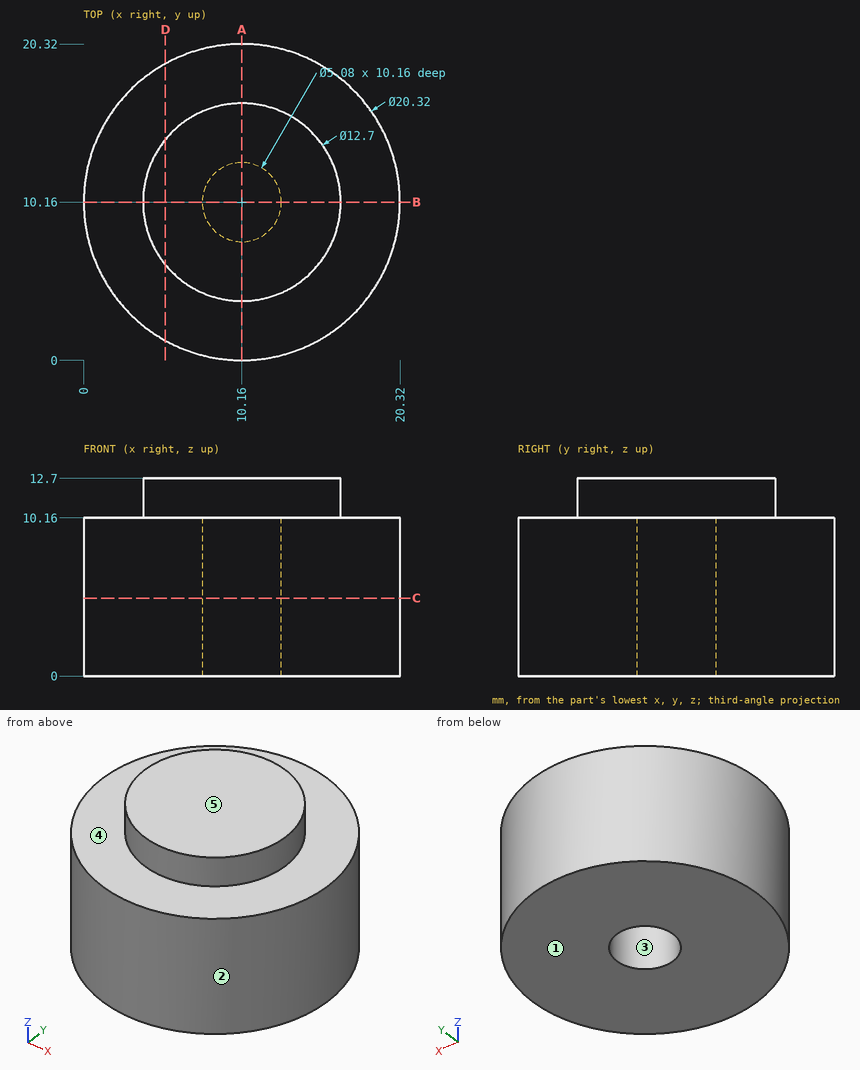
Verification items for this drawing (mm, ordinates from the low corner). A direction names the side the tool comes from. Give positions to 0.01 mm unless a question says otherwise; leave off trailing zeros. Write each loop counter-clockwise with the first axis right and the second up, starting at its lowest first coordinate (ties: lowest second). Pieces come first, ordered by that corner, then holes. Notation, with made-up numbers: (-21.75, -13) -> (-13.75, -13) arc R27 cw to (-13.75, 6) -> close; hole circle Ø8 at (67, 65.25). An arc over 180 degrees is marked (long way). Write item = value, one per line.
Item 1: Scan lines: probe 1 along Y at (x, z) = (10.16, 7.75); probe 2 along X at (y, z) = (10, 1.25); probe 3 along Z at (x, y) = (8.75, 19.5). Record each from-to range of solid material in increasing order. Write a range as from..to.
Output:
probe_1 = 0..7.62, 12.7..20.32
probe_2 = 0..7.63, 12.69..20.32
probe_3 = 0..10.16
Item 2: Sectioned sample at C-C on z = 5. Record the boundary of the cut face in (x, y).
Output:
outline = circle Ø20.32 at (10.16, 10.16); hole circle Ø5.08 at (10.16, 10.16)
Item 3: Sectioned sample at A-A on x = 10.16. Record the boundary of the cut face in (y, z).
Output:
outline = (0, 0) -> (7.62, 0) -> (7.62, 10.16) -> (12.7, 10.16) -> (12.7, 0) -> (20.32, 0) -> (20.32, 10.16) -> (16.51, 10.16) -> (16.51, 12.7) -> (3.81, 12.7) -> (3.81, 10.16) -> (0, 10.16) -> close
Item 4: Gauge pin test, flat ends, axial feed: pin 1 (4.5 mm diameter, centred on x = 10.16, y = 10.16, fed in from -Z); pin 2 (3 mm diameter, centred on x = 7.5, z = 6.5, fed in from -Y); pin 3 (2 mm diameter, centred on y = 14, z = 9.5, fed in from +X) (3 decimals). Record the tip position at first contact, or that the pin passes through.
Output:
pin_1 = 10.16
pin_2 = 0.07
pin_3 = 19.915
Item 5: Release check for a two-part mould opening along Y. For the marked faces 1, 2 and 3 record: +Y half, -Y half, draft (parallel to the pull), parting line (faces both ways), or undercut.
Output:
face_1 = draft
face_2 = parting line
face_3 = undercut
Item 6: Sectioned sample at D-D on x = 5.25. Record the boundary of the cut face in (y, z).
Output:
outline = (1.27, 0) -> (19.05, 0) -> (19.05, 10.16) -> (14.19, 10.16) -> (14.19, 12.7) -> (6.13, 12.7) -> (6.13, 10.16) -> (1.27, 10.16) -> close
Item 7: Tool access check on the marked faces 4 and 5. Record the directions out of +Z, -Z, +X, -X, +Y, -Y that give a thin tool (end or side, any length) a straight path to the whole face; none if there is none.
Output:
face_4 = +Z
face_5 = +Z, +X, -X, +Y, -Y
